Source: three-view drawing plus pictorial views. Frame: mm from the lowest corner of the part. A direction names the side the tool comes from. Give positions to 0.01 mm unless a question says otherwise; leave off trailing zeros. Order: outer loops, then holes, each group sorted by start corner. A loop starts at its lowest first (then second) coordinate and runs counter-clockwise, first axis right, second up.
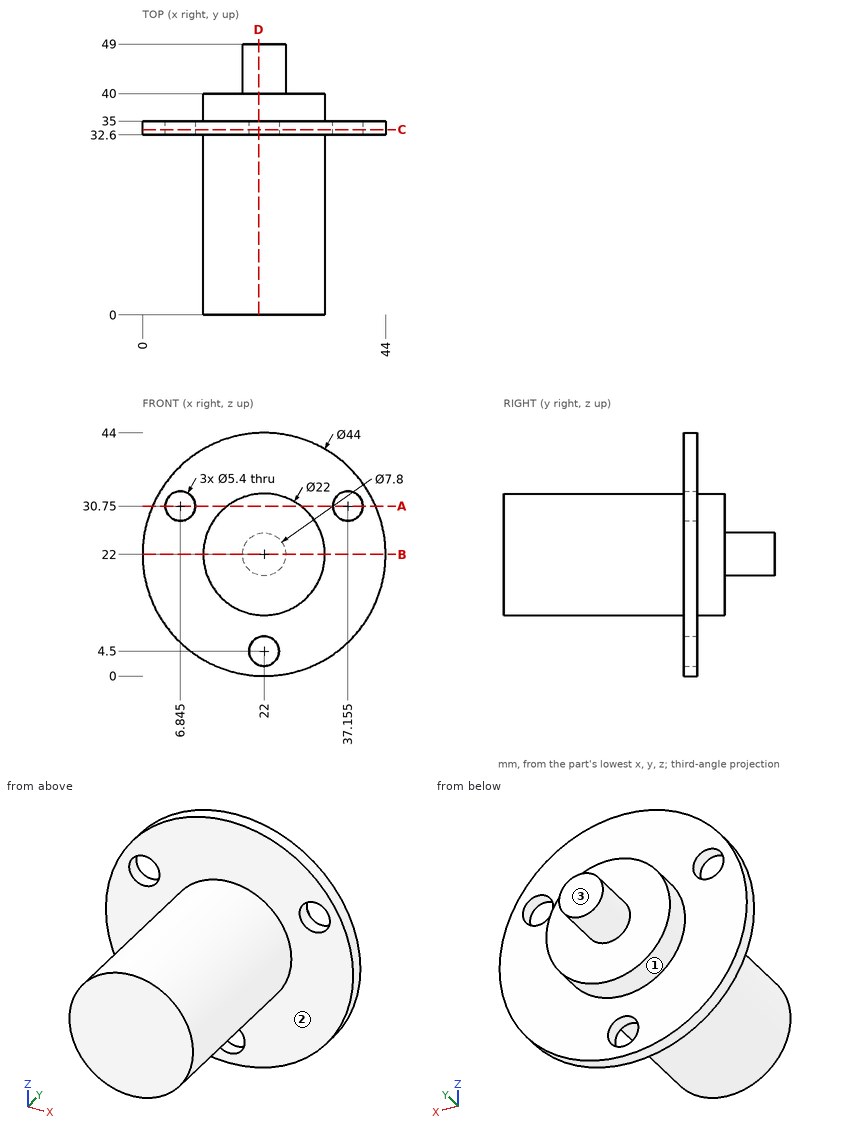
(1) Section B-B, the plane z = 22. Return loops of the section in (x, y), plus the area to 3 significant figures.
(2) Section A-A, the plane z = 30.75. Return loops of the section in (x, y) (1 decimal).
(3) Access query for the marked faces 1, 2 and 3. Directions: +Z, -Z, +X, -X, +Y, -Y. A direction counts if a zero-diameter tool reaches every point of the face in a straight line with its end or side. Return the directions, or none.
(4) Line query: line 1 along X through (y, z) = (33.9, 30.75) (1 decimal); line 2 along Z through (x, y) = (22, 33.8); line 3 along Y through (x, z) = (19, 26). Output: solid intervals per line, ascending.
(5) Section D-D, the plane x = 21. Return loops of the section in (y, z) (1 decimal).
(6) Section C-C, the plane y = 33.5. Count the separate pieces of the cut face and the enclosed holes in it, plus the area to 3 significant figures.
(7) Pin query (flat end, axial travel): pin 1 Ø10 at (x, z) = (5, 10.5) entering from -Y; pin 2 Ø6 at (y, z) = (38.5, 38.5) entering from +X; pin 3 Ø8 at (x, y) = (24.5, 34.5) entering from -Z; pin 4 Ø3 at (x, y) = (24.5, 19) entering from +Z. Return the tip coordinate at first contact, or that it passes through.
Checks:
1. outline: (0, 32.6) - (11, 32.6) - (11, 0) - (33, 0) - (33, 32.6) - (44, 32.6) - (44, 35) - (33, 35) - (33, 40) - (25.9, 40) - (25.9, 49) - (18.1, 49) - (18.1, 40) - (11, 40) - (11, 35) - (0, 35) - close
1. area: 1,000 mm2
2. outline: (1.8, 32.6) - (4.1, 32.6) - (4.1, 35) - (1.8, 35) - close; (9.5, 32.6) - (15.3, 32.6) - (15.3, 0) - (28.7, 0) - (28.7, 32.6) - (34.5, 32.6) - (34.5, 35) - (28.7, 35) - (28.7, 40) - (15.3, 40) - (15.3, 35) - (9.5, 35) - close; (39.9, 32.6) - (42.2, 32.6) - (42.2, 35) - (39.9, 35) - close
3. face 1: +Y
3. face 2: -Y
3. face 3: +Z, -Z, +X, -X, +Y
4. line 1: x = 1.8 to 4.1, 9.5 to 34.5, 39.9 to 42.2
4. line 2: z = 0 to 1.8, 7.2 to 44
4. line 3: y = 0 to 40
5. outline: (0, 11) - (32.6, 11) - (32.6, 7) - (35, 7) - (35, 11) - (40, 11) - (40, 18.2) - (49, 18.2) - (49, 25.8) - (40, 25.8) - (40, 33) - (35, 33) - (35, 44) - (32.6, 44) - (32.6, 33) - (0, 33) - close; (32.6, 0) - (35, 0) - (35, 2) - (32.6, 2) - close
6. separate pieces: 1
6. enclosed holes: 3
6. area: 1,450 mm2
7. pin 1: stops at y = 32.6
7. pin 2: passes through
7. pin 3: stops at z = 0
7. pin 4: stops at z = 32.95
